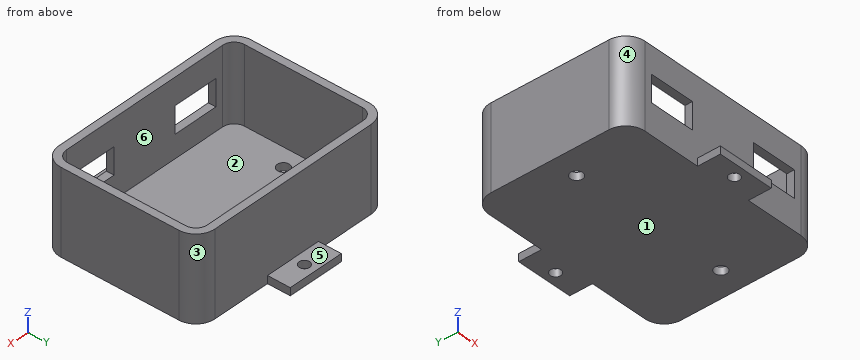
from build123d import *

# Parameters (mm, degrees)
PAD_DEPTH       = 20
THICKNESS_T     = 2
SKETCH001_W     = 15
SKETCH001_H     = 2
PAD001_DEPTH    = 6
SKETCH002_R     = 1.4
POCKET_DEPTH    = 2.001
SKETCH003_W     = 15
SKETCH003_H     = 2
PAD002_DEPTH    = 6
SKETCH004_R     = 1.4
POCKET001_DEPTH = 22.001
SKETCH005_R     = 1.6
POCKET002_DEPTH = 22.001
SKETCH006_W     = 12
SKETCH006_H     = 7
POCKET003_DEPTH = 2


with BuildPart() as part:
    # Sketch → Pad (new body)
    with BuildSketch(Plane.XY):
        with BuildLine():
            Line((0, 37), (46, 37))
            ThreePointArc((49, 34), (48.1213203436, 36.1213203436), (46, 37))
            Line((49, 34), (49, 3))
            ThreePointArc((46, 0), (48.1213203436, 0.8786796564), (49, 3))
            Line((46, 0), (0, 0))
            ThreePointArc((-3, 3), (-2.1213203436, 0.8786796564), (0, 0))
            Line((-3, 3), (-3, 34))
            ThreePointArc((0, 37), (-2.1213203436, 36.1213203436), (-3, 34))
        make_face()
    extrude(amount=PAD_DEPTH)

    # Thickness
    thickness_openings = [part.faces().sort_by_distance(p)[0] for p in [
        (23, 18.5, 20),
    ]]
    offset(amount=THICKNESS_T, openings=thickness_openings, kind=Kind.INTERSECTION)

    # Sketch001 → Pad001 (new body)
    with BuildSketch(Plane(origin=(0, 39, 0), x_dir=(-1, 0, 0), z_dir=(0, 1, 0))):
        with Locations((-23, -1)):
            Rectangle(SKETCH001_W, SKETCH001_H)
    extrude(amount=PAD001_DEPTH)

    # Sketch002 → Pocket (cut, through all)
    with BuildSketch(Plane.XY):
        with Locations((23, 42)):
            Circle(SKETCH002_R)
    extrude(amount=-POCKET_DEPTH, mode=Mode.SUBTRACT)

    # Sketch003 → Pad002 (new body)
    with BuildSketch(Plane.XZ.offset(2)):
        with Locations((23, -1)):
            Rectangle(SKETCH003_W, SKETCH003_H)
    extrude(amount=PAD002_DEPTH)

    # Sketch004 → Pocket001 (cut, through all)
    with BuildSketch(Plane(origin=(0, 0, -2), x_dir=(1, 0, 0), z_dir=(0, 0, -1))):
        with Locations((23, 5)):
            Circle(SKETCH004_R)
    extrude(amount=-POCKET001_DEPTH, mode=Mode.SUBTRACT)

    # Sketch005 → Pocket002 (cut, through all)
    with BuildSketch(Plane(origin=(0, 0, -2), x_dir=(1, 0, 0), z_dir=(0, 0, -1))):
        with Locations((2, -17.739397)):
            Circle(SKETCH005_R)
        with Locations((44, -17.314964)):
            Circle(SKETCH005_R)
    extrude(amount=-POCKET002_DEPTH, mode=Mode.SUBTRACT)

    # Sketch006 → Pocket003 (cut)
    with BuildSketch(Plane.XZ.offset(2)):
        with Locations((8, 9.5)):
            Rectangle(SKETCH006_W, SKETCH006_H)
        with Locations((38, 9.5)):
            Rectangle(SKETCH006_W, SKETCH006_H)
    extrude(amount=-POCKET003_DEPTH, mode=Mode.SUBTRACT)


solid = part.part
Input: part model. Units: mm. Frame: model coordinates. Face numbers are marked on the shaded views. A direction names the side the tool comes from. Coordinates: 2 decimals unless noted, no trailing zeros. Write each loop counter-clockwise with the first axis right and the second up, starting at its lowest first coordinate (ties: lowest second). Pieces come first, ordered by that corner, then holes. Notation, with made-up numbers: M 9,81.25 L 43,81.25 A26 cw 43,100.25 Z; hole C 6,76.5 d5. An arc over 180 degrees is marked long. Answer as a JSON object with one key per item and string values. Group by question number.
(1) Ray query, line 1 along Y through (x, z) = (23, -0.85); line 2 along Y through (x, z) = (17, 15.5); line 3 along X through (y, z) = (24, 10.5). Return the intervals inside material, ascending. Write a range as [from, to].
(2) Section A-A on y = -5. Output: boundary loops of the cut face in (x, z), plus the area to 3 significant figures.
(3) Mould query, pull axis X, two halves, no side actions, for the marked faces 1, 2 and 3. Classes: pulls with the +X half, pulls with the -X half, needs draft (parallel to the pull), parting line crosses it, or undercut.
(4) Section B-B on x = 33.5. Output: boundary loops of the cut face in (y, z), plus the area to 3 significant figures.
(5) Contact query for flat-ended pins moving along their axis: P1, Ø10, axis at x = 13.5, z = 14, coming from the -Y side; P2, Ø0.6, axis at y = -4.5, z = -0.5, coming from the +X side; P3, Ø1.6, axis at y = 42, z = -1.5, coming from the -X side. Output: stop coordinate, or through.
(6) Section C-C on x = 23. Output: boundary loops of the cut face in (y, z), plus the area to 3 significant figures.
(7) Section D-D on y = 13. Output: boundary loops of the cut face in (x, z).
(8) Set-up query: the marked faces 4, 5 and 6. Return all of +Z, -Z, +X, -X, +Y, -Y with unobstructed straight access to the full face (end or side cutting, diameter ignored); none if empty.
Result set:
{
 "1": {"line 1": "y = [-8, -6.4], [-3.6, 40.6], [43.4, 45]", "line 2": "y = [-2, 0], [37, 39]", "line 3": "x = [-5, -3], [49, 51]"},
 "2": {"outline": "M 15.5,-2 L 21.6,-2 L 21.6,0 L 15.5,0 Z; M 24.4,-2 L 30.5,-2 L 30.5,0 L 24.4,0 Z", "area": "24.4 mm2"},
 "3": {"face 1": "needs draft", "face 2": "undercut", "face 3": "pulls with the +X half"},
 "4": {"outline": "M -2,-2 L 39,-2 L 39,20 L 37,20 L 37,0 L 0,0 L 0,6 L -2,6 Z; M -2,13 L 0,13 L 0,20 L -2,20 Z", "area": "148 mm2"},
 "5": {"P1": "stops at y = -2", "P2": "stops at x = 30.5", "P3": "stops at x = 15.5"},
 "6": {"outline": "M -8,-2 L -6.4,-2 L -6.4,0 L -8,0 Z; M -3.6,-2 L 40.6,-2 L 40.6,0 L 39,0 L 39,20 L 37,20 L 37,0 L 0,0 L 0,20 L -2,20 L -2,0 L -3.6,0 Z; M 43.4,-2 L 45,-2 L 45,0 L 43.4,0 Z", "area": "175 mm2"},
 "7": {"outline": "M -5,-2 L 51,-2 L 51,20 L 49,20 L 49,0 L -3,0 L -3,20 L -5,20 Z"},
 "8": {"face 4": "+Z, -Z, -X, -Y", "face 5": "+Z, +X, -X, +Y", "face 6": "+Z"}
}
